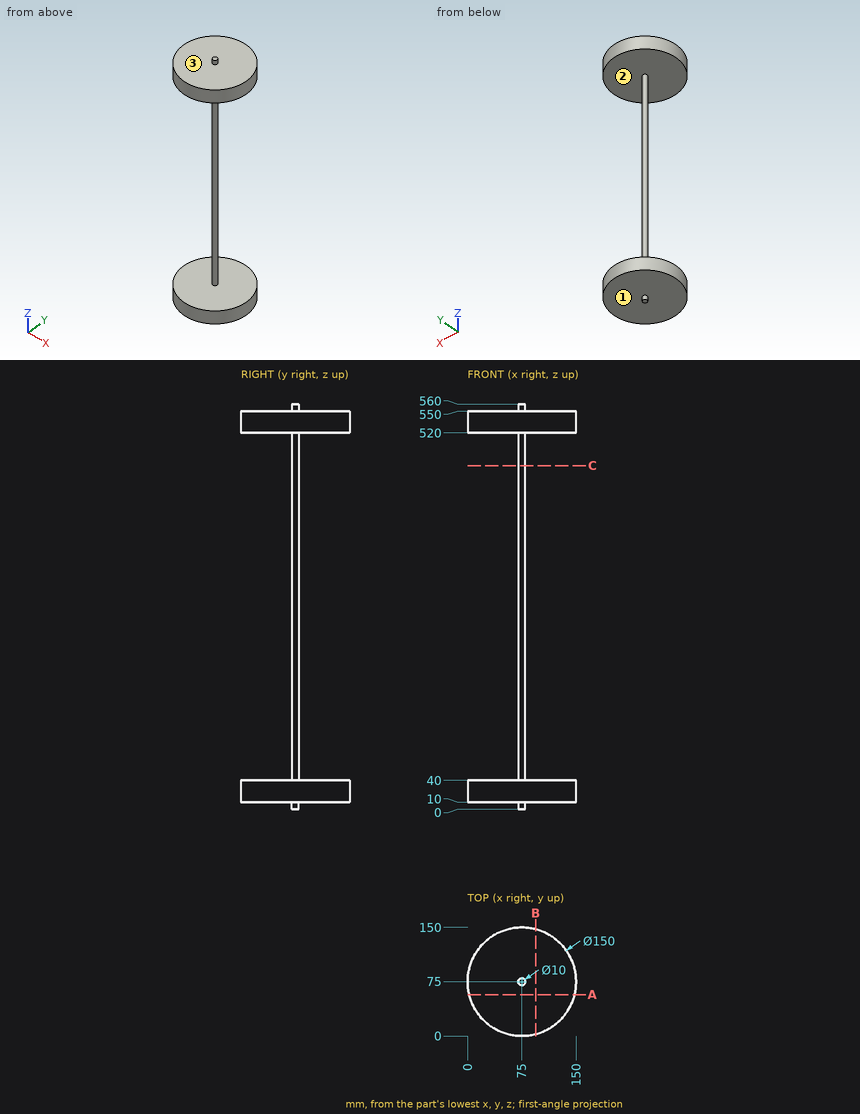
Geometry: see drawing. Coordinates: mm, zero at the bounding-box minimum. Give positions to 0.01 mm unless a question says otherwise; leave off trailing zeros. Write each loop counter-clockwise with the first axis right and the second up, starting at its lowest first coordinate (ties: lowest second). Pieces come first, ordered by that corner, then holes. Notation, with made-up numbers: (-3, 28) -> (21, 28) arc R25 cw to (21, 64) -> close; hole circle Ø10 at (0, -25). An arc over 180 degrees is marked (long way). Use one line per item in the form item = value. Start each with the question number.
1) Pin query (flat end, axial travel): pin 1 (12 mm diameter, centred on x = 115.5, y = 91, fed in from +Z); pin 2 (1.5 mm diameter, centred on x = 65.5, y = 111, fed in from -Z). Return the tip coordinate at first contact, or that it passes through.
2) Section query A-A on y = 57. Return the cut outline in (x, z).
3) Draft query along Z for the marked faces 1, 2 and 3. Return one class per face: pulls with the +Z half, pulls with the -Z half, needs draft (parallel to the pull), parting line crosses it, or undercut.
4) Section query C-C on z = 475. Return the cut outline in (x, y), then the cut area to 3 significant figures.
5) Section query B-B on x = 94. Return the cut outline in (y, z).
6) Ray query, probe 1 along Z at (x, y) = (112, 24); probe 2 along Y at (x, z) = (78, 396.5); probe 3 along X at (y, z) = (82, 535). Return the intervals inside material, ascending. Write a range as from..to.
Outcome:
q1.pin_1 = 550
q1.pin_2 = 10
q2.outline = (2.19, 10) -> (147.81, 10) -> (147.81, 40) -> (2.19, 40) -> close; (2.19, 520) -> (147.81, 520) -> (147.81, 550) -> (2.19, 550) -> close
q3.face_1 = pulls with the -Z half
q3.face_2 = undercut
q3.face_3 = pulls with the +Z half
q4.outline = circle Ø10 at (75, 75)
q4.area = 78.5 mm^2
q5.outline = (2.45, 10) -> (147.55, 10) -> (147.55, 40) -> (2.45, 40) -> close; (2.45, 520) -> (147.55, 520) -> (147.55, 550) -> (2.45, 550) -> close
q6.probe_1 = 10..40, 520..550
q6.probe_2 = 71..79
q6.probe_3 = 0.33..149.67
